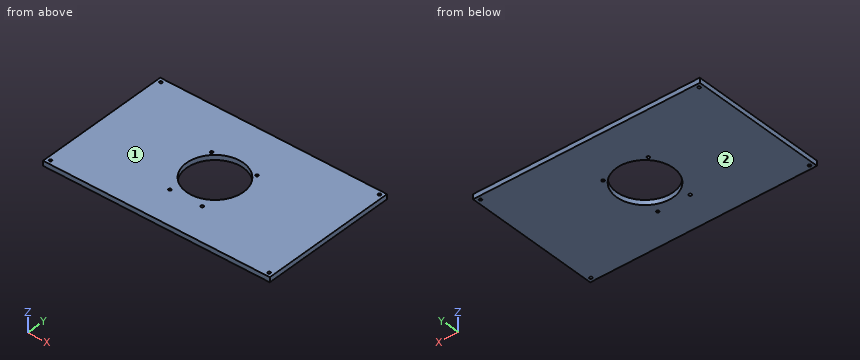
```python
from build123d import *

# Parameters (mm, degrees)
SKETCH_W      = 280
SKETCH_H      = 170
SKETCH_R      = 1.7
PAD_DEPTH     = 6
SKETCH002_R   = 35.14
SKETCH002_R_2 = 1.7
POCKET_DEPTH  = 6.001


with BuildPart() as part:
    # Sketch → Pad (new body)
    with BuildSketch(Plane.XY):
        Rectangle(SKETCH_W, SKETCH_H)
        with Locations((-135, 80)):
            Circle(SKETCH_R, mode=Mode.SUBTRACT)
        with Locations((-135, -80)):
            Circle(SKETCH_R, mode=Mode.SUBTRACT)
        with Locations((135, 80)):
            Circle(SKETCH_R, mode=Mode.SUBTRACT)
        with Locations((135, -80)):
            Circle(SKETCH_R, mode=Mode.SUBTRACT)
    extrude(amount=PAD_DEPTH)

    # Sketch002 (on Face10 of Pad) → Pocket (cut, through all)
    with BuildSketch(Plane.XY.offset(6)):
        Circle(SKETCH002_R)
        with Locations((-28, 28)):
            Circle(SKETCH002_R_2)
        with Locations((28, 28)):
            Circle(SKETCH002_R_2)
        with Locations((-20, -42)):
            Circle(SKETCH002_R_2)
        with Locations((20, -42)):
            Circle(SKETCH002_R_2)
    extrude(amount=-POCKET_DEPTH, mode=Mode.SUBTRACT)


solid = part.part
```
Here's how the part is built. I have some questions about the finished solid (model axes, mm). Face numbers are marked on the shaded views. Round coordinates to 2 decimals unless told otherwise and drop trailing zeros. Order: outer loops, then holes, each group sorted by start corner. A loop starts at its lowest first (then second) coordinate and runs counter-clockwise, first axis right, second up. Notation, with made-up numbers: (-7.75, -26.75) -> (7.25, -26.75) arc R5 ccw to (7.25, -20.75) -> close; hole circle Ø7 at (-31.5, 64). An arc over 180 degrees is marked (long way). Use a Markdown table: item, result. Add a question column.
(1) For pin 1 Ø2 at (x, y) = (20, -42) entering from +Z; pin 2 Ø5 at (x, y) = (-30.5, 53.5) entering from -Z, each with a flat end and sliding along its axis, tell me the tip position at first contact or that it passes through.
(2) If we mould it in two halves opening along Z, with no side actions, what happens to the marked faces 1 and 2? For each: released by +Z, released by -Z, zero draft, split by the parting line, or undercut.
(3) Suppose I cut it at B-B, the plane z = 3.45. Count the separate pieces of the cut face and the enclosed holes in it, and give its area (3 significant figures).
(4) Suppose I cut it at C-C, the plane y = 15. Please give me the cut outline in (x, z), and give its area (3 significant figures).
(5) Suppose I cut it at A-A, the plane x = 0. Please give me the cut outline in (y, z).
(6) I need wall thicknesses on line 1 along X through (y, z) = (-80, 2.9); line 2 along Y through (x, z) = (-20, 3.4); line 3 along Y through (x, z) = (-27.5, 2.25). Which ranges of each line are inside material? Lowest first, please.
Verdict:
| question | item | result |
|---|---|---|
| 1 | pin 1 | through |
| 1 | pin 2 | z = 0 |
| 2 | face 1 | released by +Z |
| 2 | face 2 | released by -Z |
| 3 | separate pieces | 1 |
| 3 | enclosed holes | 9 |
| 3 | area | 43,600 mm2 |
| 4 | outline | (-140, 0) -> (-31.78, 0) -> (-31.78, 6) -> (-140, 6) -> close; (31.78, 0) -> (140, 0) -> (140, 6) -> (31.78, 6) -> close |
| 4 | area | 1,300 mm2 |
| 5 | outline | (-85, 0) -> (-35.14, 0) -> (-35.14, 6) -> (-85, 6) -> close; (35.14, 0) -> (85, 0) -> (85, 6) -> (35.14, 6) -> close |
| 6 | line 1 | -140 to -136.7, -133.3 to 133.3, 136.7 to 140 |
| 6 | line 2 | -85 to -43.7, -40.3 to -28.89, 28.89 to 85 |
| 6 | line 3 | -85 to -21.88, 21.88 to 26.38, 29.62 to 85 |
